Design review of the part built by this model. Coordinates are the model's own, in mm. A direction names the side the tool comes from. Give positions to 0.01 mm unless a question says otherwise; leave off trailing zeros. Order: outer loops, then holes, each group sorted by start corner. A loop starts at its lowest first (then second) coordinate and runs counter-clockwise, first axis right, second up. Notation, with made-up numbers: (49.5, 61.5) -> (73.5, 61.5) arc R28 cw to (73.5, 82.5) -> close; hole circle Ø5 at (51, 68.25). An arc over 180 degrees is marked (long way). Return JSON: item names as keys, results as strings.
```python
from build123d import *
from build123d.topology import SkipClean

# Parameters (mm, degrees)
CUT_EXTRUDE2_DEPTH = 3.5
SKETCH7_R          = 1.2
CUT_EXTRUDE6_DEPTH = 7
SKETCH3_R          = 5.3
CUT_EXTRUDE7_DEPTH = 24.098268333
CUT_EXTRUDE8_START = 3
SKETCH8_R          = 2.5
CUT_EXTRUDE8_DEPTH = 22.371910061


with BuildPart() as part:
    # Sketch1 → Revolve1 (revolve)
    with SkipClean():  # the faces are left unmerged after this step: merging them gives an invalid solid
        with BuildSketch(Plane.XY):
            with BuildLine():
                ThreePointArc((0, 14.4), (-10.182337649, 10.182337649), (-14.4, 0))
                Line((-14.4, 0), (0, 0))
                Line((0, 0), (0, 14.4))
            make_face()
            with BuildLine():
                Line((0, 14.4), (0, 0))
                Line((0, 0), (14.4, 0))
                ThreePointArc((14.4, 0), (10.182337649, 10.182337649), (0, 14.4))
            make_face()
        revolve(axis=Axis((0, -1000, 0), (0, 1, 0)))
    add(part.part.scale(1), mode=Mode.REPLACE)  # the faces are merged on a copy

    # Sketch2 → Cut-Extrude2 (cut)
    with BuildSketch(Plane.XZ):
        Polygon((4.936344802, -8.55), (9.872689603, 0), (4.936344802, 8.55), (-4.936344802, 8.55), (-9.872689603, 0), (-4.936344802, -8.55), align=None)
    extrude(amount=-CUT_EXTRUDE2_DEPTH, mode=Mode.SUBTRACT)

    # Sketch7 → Cut-Extrude6 (cut)
    with BuildSketch(Plane.XZ):
        with Locations((-9.526279442, 5.5)):
            Circle(SKETCH7_R)
        with Locations((9.526279442, 5.5)):
            Circle(SKETCH7_R)
        with Locations((0, -11)):
            Circle(SKETCH7_R)
    extrude(amount=-CUT_EXTRUDE6_DEPTH, mode=Mode.SUBTRACT)

    # Sketch3 → Cut-Extrude7 (cut, through all)
    with BuildSketch(Plane.XZ.offset(-3.5)):
        Circle(SKETCH3_R)
    extrude(amount=-CUT_EXTRUDE7_DEPTH, mode=Mode.SUBTRACT)

    # Sketch8 → Cut-Extrude8 (cut, through all)
    with BuildSketch(Plane(origin=(0, 0, 0), x_dir=(1, 0, 0), z_dir=(0, 1, 0)).offset(CUT_EXTRUDE8_START)):
        with Locations(Location((-9.526279442, -5.5, 0), (0, 0, 41.478340955))):
            Circle(SKETCH8_R)
        with Locations(Location((0, 11, 0), (0, 0, 116.349338557))):
            Circle(SKETCH8_R)
        with Locations(Location((9.526279442, -5.5, 0), (0, 0, 138.521659045))):
            Circle(SKETCH8_R)
    extrude(amount=CUT_EXTRUDE8_DEPTH, mode=Mode.SUBTRACT)


solid = part.part
```
Item 1: Mouldability with a two-part tool opening along Z and no side actions: class faces 4 (the face through (7, 0, 6)), 5 (the face through (-7.37, 1.726, 4.335)), 6 (the face through (0, 2, -8.55)) as released by +Z, released by -Z, zero draft, split by the parting line, or undercut.
Result set:
{"face 4": "zero draft", "face 5": "undercut", "face 6": "undercut"}
Item 2: Add section C-C (y = 8). Give the boundary of the cut face in (x, z).
Result set:
{"outline": "(-11.36, 3.8) arc R11.97 ccw to (-2.39, -11.73) arc R2.5 cw (long way) to (2.39, -11.73) arc R11.97 ccw to (11.36, 3.8) arc R2.5 cw (long way) to (8.97, 7.94) arc R11.97 ccw to (-8.97, 7.94) arc R2.5 cw (long way) to start; hole circle Ø10.6 at (0, 0)"}
Item 3: Machinability: for faces 1 (the face through (7.37, 1.726, -4.335)), 2 (the face through (4.896, 8.375, -2.03)), 3 (the face through (-1, 3, -12)), which of the approach directions +Z, -Z, +X, -X, +Y, -Y give a long, thin tool a straight path to every point of the face, cutting with its end or side? Answer none if there is none.
Result set:
{"face 1": "-Y", "face 2": "+Y, -Y", "face 3": "+Y"}
Item 4: Add section D-D (x = 11.5). Give the boundary of the cut face in (y, z).
Result set:
{"outline": "(0, -8.67) arc R8.67 ccw to (7.71, 3.97) -> (3, 3.97) -> (3, 7.03) -> (5.06, 7.03) arc R8.67 ccw to (0, 8.67) -> close"}
Item 5: Add section B-B (z = -1). Give the boundary of the cut face in (x, y).
Result set:
{"outline": "(-14.37, 0) -> (-9.3, 0) -> (-9.3, 3.5) -> (-5.2, 3.5) -> (-5.2, 13.39) arc R14.37 ccw to start; (5.2, 3.5) -> (9.3, 3.5) -> (9.3, 0) -> (14.37, 0) arc R14.37 ccw to (5.2, 13.39) -> close"}
Item 6: Wall thickness on L1, parallel to X at y = 4.75, z = 5.5; L2, parallel to Z at x = 0, y = 3.75; L3, parallel to Z at x = 0, y = 8.5: over which ranges is each line inside the solid? List them lowest first. Write a range as [from, to].
Result set:
{"L1": "x = [-12.43, -12.03], [-7.03, 7.03], [12.03, 12.43]", "L2": "z = [-13.9, -13.5], [-8.5, -5.3], [5.3, 13.9]", "L3": "z = [-8.5, -5.3], [5.3, 11.62]"}
Item 7: Add section A-A (x = 0). Give the boundary of the cut face in (y, z).
Result set:
{"outline": "(0, -14.4) arc R14.4 ccw to (5.01, -13.5) -> (3, -13.5) -> (3, -12.2) -> (0, -12.2) -> close; (0, -9.8) -> (3, -9.8) -> (3, -8.55) -> (0, -8.55) -> close; (0, 8.55) -> (3.5, 8.55) -> (3.5, 5.3) -> (13.39, 5.3) arc R14.4 ccw to (0, 14.4) -> close; (3.5, -8.5) -> (11.62, -8.5) arc R14.4 ccw to (13.39, -5.3) -> (3.5, -5.3) -> close"}
Item 8: For pin 1 (3 mm diameter, centred on x = -1.5, y = 2, fed in from +Z); pin 2 (4 mm diameter, centred on x = 7, z = 8.5, fed in from +Y); pin 3 (14 mm diameter, centred on x = 0, z = 0, fed in from -Y); pin 4 (3 mm diameter, centred on x = 9.53, z = 5.5, fed in from -Y), all flat-tipped, find the tip position at first contact; note any pin that passes through.
Result set:
{"pin 1": "stops at z = 14.37", "pin 2": "stops at y = 11.23", "pin 3": "stops at y = 3.5", "pin 4": "stops at y = 0"}
